from build123d import *

# Parameters (mm, degrees)
F0_W     = 152.4
F0_H     = 254
F1_DEPTH = 76.2
F3_DEPTH = 152.4
F5_DEPTH = 254.001
F7_DEPTH = 152.401
F9_DEPTH = 3.175


with BuildPart() as f1:
    # F0 (on Top) → F1 (new body)
    with BuildSketch(Plane.XY):
        with Locations((76.2, 127)):
            Rectangle(F0_W, F0_H)
    extrude(amount=F1_DEPTH)

    # F2 (on face) → F3 (cut, through all)
    with BuildSketch(Plane.YZ.offset(152.4)):
        Polygon((0, 76.2), (0, 0), (254, 76.2), align=None)
    extrude(amount=-F3_DEPTH, mode=Mode.SUBTRACT)

    # F4 (on face) → F5 (cut, through all)
    with BuildSketch(Plane(origin=(0, 254, 0), x_dir=(-1, 0, 0), z_dir=(0, 1, 0))):
        Polygon((0, 76.2), (-152.4, 76.2), (0, 0), align=None)
    extrude(amount=-F5_DEPTH, mode=Mode.SUBTRACT)

    # F6 (on face) → F7 (cut, through all)
    with BuildSketch(Plane.YZ.offset(152.4)):
        Polygon((254, 0), (254, 76.2), (177.8, 0), align=None)
    extrude(amount=-F7_DEPTH, mode=Mode.SUBTRACT)

    # F8 (on face) → F9 (join)
    with BuildSketch(Plane(origin=(0, 88.9, -88.9), x_dir=(-1, 0, 0), z_dir=(0, 0.7071067812, -0.7071067812))):
        Polygon((-152.4, 233.4866591478), (0, 125.723585695), (0, 233.4866591478), align=None)
        Polygon((-152.4, 125.7235856949), (0, 125.7235856949), (-152.4, 233.4866591478), align=None)
    extrude(amount=F9_DEPTH)


solid = f1.part
Could you check a few things on this model? Use its own coordinates, in mm. A direction names the side the tool comes from. Round coordinates to 2 decimals unless told otherwise and drop trailing zeros. Order: outer loops, then holes, each group sorted by start corner. A loop starts at its lowest first (then second) coordinate and runs counter-clockwise, first axis right, second up.
(1) Imagine slicing it at C-C (y = 207.5). Write out the boundary of the cut face in (x, z).
Response values:
outline: (0, 25.21) - (152.4, 25.21) - (152.4, 62.25) - (124.5, 62.25) - (59.4, 29.7) - (0, 29.7) - close
(2) Imagine slicing it at A-A (x = 102). Write out the boundary of the cut face in (y, z).
Response values:
outline: (0, 0) - (177.8, 0) - (180.05, -2.25) - (256.25, 73.95) - (254, 76.2) - (228.8, 51) - (170, 51) - close
(3) I'm going to push flat-ended pins straight in: pin 1 (2 mm diameter, centred on y = 198.5, z = 29.5, fed in from -X); pin 2 (6 mm diameter, centred on x = 117, y = 167, fed in from +Z); pin 3 (12 mm diameter, centred on x = 36, z = 14, fed in from +Y). Where does each tip first touch, or does it pass through?
Response values:
pin 1: stops at x = 57
pin 2: stops at z = 51
pin 3: stops at y = 202.29
(4) Please list where these lines run through material, in increasing order: line 1 along Y through (x, z) = (127, 67); line 2 along Z through (x, y) = (97, 205); line 3 along Z through (x, y) = (24.5, 93).
Response values:
line 1: y = 244.8 to 249.29
line 2: z = 22.71 to 48.5
line 3: z = 0 to 12.25
(5) Which directions (+Z, -Z, +X, -X, +Y, -Y) give clear straight access to the entire face, cutting with the end or side of a thin tool? Please do faces 1 (the flat face through (152.4, 151, 27)), 2 (the flat face through (75, 90, 0)), 3 (the flat face through (43.4, 233.4, 55.6)).
Response values:
face 1: +Z, -Z, +X, +Y, -Y
face 2: -Z, +X, -X, -Y
face 3: +Z, -X, -Y
(6) Imagine slicing it at B-B (z = 58.5). Write out the boundary of the cut face in (x, y).
Response values:
outline: (0, 236.3) - (117, 236.3) - (117, 195) - (152.4, 195) - (152.4, 240.79) - (0, 240.79) - close
(7) Imagine slicing it at D-D (x = 40.5). Write out the boundary of the cut face in (y, z), plus the area to 3 significant figures.
Response values:
outline: (0, 0) - (177.8, 0) - (180.05, -2.25) - (256.25, 73.95) - (254, 76.2) - (198.05, 20.25) - (67.5, 20.25) - close
area: 3,460 mm2
